Autodesk Inventor part; units mm, degrees
ref_plane "YZ Plane" through (0, 0, 0) normal (1, 0, 0) x (0, 1, 0)
ref_plane "XZ Plane" through (0, 0, 0) normal (0, 1, 0) x (-1, 0, 0)
ref_plane "XY Plane" through (0, 0, 0) normal (0, 0, 1) x (1, 0, 0)
sketch "Skizze1" plane through (0, 0, 0) normal (0, 0, 1) x (1, 0, 0)
  line L0 (0, 12.3) -> (8.8, 12.3)
  line L1 (0, 12.3) -> (0, 0)
  line L2 (0, 0) -> (8.8, 0)
  line L3 (8.8, 0) -> (8.8, 12.3)
  circle A0 centre (5.18, 3.55) radius 1.25
  circle A1 centre (5.18, 3.55) radius 1.25
  line L4 (0, 12.3) -> (8.8, 12.3)
  line L5 (8.8, 12.3) -> (8.8, 0)
  line L6 (8.8, 0) -> (0, 0)
  line L7 (0, 0) -> (0, 12.3)
  dimension "d35" = 8.8
  dimension "d36" = 5.18
extrude "Extrusion1" add sketch "Skizze1" along normal blind 9.8
sketch "Skizze2" plane through (8.8, 0, 0) normal (1, 0, 0) x (0, 0, -1)
  line L0 (0, 0) -> (-9.8, 0)
  line L1 (0, 0) -> (0, 12.3)
  line L2 (0, 12.3) -> (-9.8, 12.3)
  line L3 (-4.8, 6.1) -> (0, 6.1)
  line L4 (0, 6.1) -> (0, 0)
  line L5 (0, 0) -> (-4.8, 0)
  line L6 (-4.8, 0) -> (-4.8, 6.1)
  dimension "d2" = 6.2
  dimension "d3" = 4.8
  dimension "d4" = 6.1
extrude "Extrusion2" cut sketch "Skizze2" against normal blind 9.8
sketch "Skizze3" plane through (8.8, 0, 9.8) normal (1, 0, 0) x (0, 0, -1)
  line L0 (9.8, 6.1) -> (9.8, 12.3)
  line L1 (9.8, 12.3) -> (0, 12.3)
  point P0 (9.8, 0)
  point P1 (6.1, 8.6)
  dimension "d7" = 3.7
  dimension "d8" = 3.7
hole "Hole1" at (8.8, 8.6, 3.7) direction (-1, 0, 0) diameter 2.013 end through all
sketch "Skizze4" plane through (0, 0, 9.8) normal (0, 0, 1) x (1, 0, 0)
  circle A0 centre (5.18, 3.55) radius 1.25
  circle A1 centre (5.18, 3.55) radius 1.25
extrude "Extrusion3" add sketch "Skizze4" against normal blind 5
sketch "Skizze5" plane through (0, 0, 9.8) normal (0, 0, 1) x (1, 0, 0)
  line L0 (8.8, 0) -> (0, 0)
  line L1 (8.8, 12.3) -> (8.8, 0)
  point P0 (5.2, 3.55)
  dimension "d18" = 3.6
  dimension "d19" = 3.55
hole "Hole2" at (5.2, 3.55, 9.8) direction (0, 0, -1) diameter 2.013 depth 8 tip angle 118
fillet "Rundung1" radius 0.2 1 edges at (0, 12.3, 4.9)
fillet "Rundung2" radius 0.1 18 edges at (0, 9.1, 0) (0.0586, 12.2414, 0) (4.5, 12.3, 0) (0, 6.1, 2.4) (0, 3.05, 4.8) (4.4, 0, 4.8) (4.4, 6.1, 4.8) (4.4, 6.1, 0) (8.8, 9.2, 0) (8.8, 3.05, 4.8) (8.8, 0, 7.3) (0, 0, 7.3) (8.8, 12.3, 4.9) (8.8, 6.15, 9.8) (4.4, 0, 9.8) (0, 6.05, 9.8) (0.0586, 12.2414, 9.8) (4.5, 12.3, 9.8)
sketch "Skizze6" plane through (0.1, 0, 9.7) normal (0, -1, 0) x (1, 0, 0)
  line L0 (8.6, 0.1) -> (0, 0.1)
  line L1 (-0.1, 0) -> (-0.1, -4.8)
  line L2 (8.7, -4.8) -> (8.7, 0)
  line L3 (1.699, 0.1) -> (6.901, 0.1)
  line L4 (6.901, 0.1) -> (6.901, -0.1)
  line L5 (6.901, -0.1) -> (1.699, -0.1)
  line L6 (1.699, -0.1) -> (1.699, 0.1)
  point P0 (-0.1, -9.7)
  dimension "d30" = 0.2
  dimension "d31" = 1.799
  dimension "d32" = 1.799
extrude "Extrusion4" cut sketch "Skizze6" against normal blind 12.5
properties part number "3. Leiterplattenhalter_Rechts"
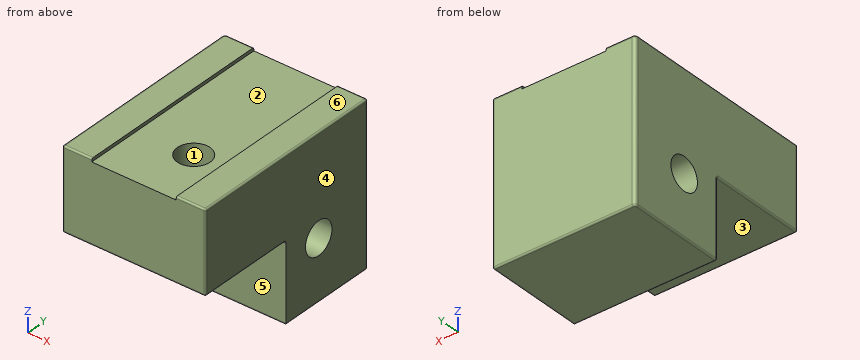
The model under review builds one solid part; all positions refer to its coordinate system, in mm. Face numbers are marked on the shaded views. A direction names the side the tool comes from. Round coordinates to 2 decimals unless told otherwise and drop trailing zeros. Order: outer loops, then holes, each group sorted by start corner. A loop starts at its lowest first (then second) coordinate and runs counter-clockwise, first axis right, second up. Notation, with made-up numbers: (12, 21.5) -> (67, 21.5) arc R19 cw to (67, 55.5) -> close; hole circle Ø1 at (-37.75, 5). An arc over 180 degrees is marked (long way). One line per item, written item: value. Start each with the question number.
Q1. Clearance check with flat-ended pins moving along their axes: pin 1 Ø4 at (x, y) = (4, 7) entering from +Z; pin 2 Ø5 at (x, z) = (5.5, 1.5) entering from -Y; pin 3 Ø4.5 at (x, y) = (2.5, 2.5) entering from -Z. State where each tip first meets the part, or that it passes through.
Q2. Machinability: for the marked faces 5 and 6, which of the approach directions +Z, -Z, +X, -X, +Y, -Y give a long, thin tool a straight path to every point of the face, cutting with its end or side? Answer none if there is none.
Q3. Take a section at C-C (y = 3.55). Write out the cut boundary in (x, z), and give its area (3 significant figures).
Q4. Take a section at A-A (x = 5.2). Write out the cut boundary in (y, z), and give its area (3 significant figures).
Q5. Take a section at B-B (z = 3.7). Write out the cut boundary in (x, y).
Q6. Mouldability with a two-part tool opening along X and no side actions: class the marked faces 1, 2, 3 and 4 as released by +X, released by -X, zero draft, split by the parting line, or undercut.
Q7. Wall thickness on line 1 (X direction, y = 3.55, z = 7.55); line 2 (Y direction, x = 2.25, z = 3.7); line 3 (Z direction, x = 3.75, y = 8.6): over which ranges is each line inside the solid? List them lowest first.
Q8. Take a section at D-D (x = 8.25). Write out the cut boundary in (y, z), and give its area (3 significant figures).
Reported:
1. pin 1: stops at z = 9.6
1. pin 2: stops at y = 6.1
1. pin 3: stops at z = 4.8
2. face 5: -Z, +X, -X, -Y
2. face 6: +Z, +X, -X, +Y, -Y
3. outline: (0, 4.9) arc R0.1 ccw to (0.1, 4.8) -> (4.19, 4.8) -> (4.19, 9.6) -> (1.8, 9.6) -> (1.8, 9.8) -> (0.1, 9.8) arc R0.1 ccw to (0, 9.7) -> close; (6.21, 4.8) -> (8.7, 4.8) arc R0.1 ccw to (8.8, 4.9) -> (8.8, 9.7) arc R0.1 ccw to (8.7, 9.8) -> (7, 9.8) -> (7, 9.6) -> (6.21, 9.6) -> close
3. area: 33.3 mm2
4. outline: (0, 4.9) arc R0.1 ccw to (0.1, 4.8) -> (2.54, 4.8) -> (2.54, 9.6) -> (0, 9.6) -> close; (4.56, 4.8) -> (6, 4.8) arc R0.1 cw to (6.1, 4.7) -> (6.1, 0.1) arc R0.1 ccw to (6.2, 0) -> (12.2, 0) arc R0.1 ccw to (12.3, 0.1) -> (12.3, 9.6) -> (4.56, 9.6) -> close; hole circle Ø2.01 at (8.6, 3.7)
4. area: 76.0 mm2
5. outline: (0, 6.2) arc R0.1 ccw to (0.1, 6.1) -> (8.8, 6.1) -> (8.8, 7.59) -> (0, 7.59) -> close; (0, 9.61) -> (8.8, 9.61) -> (8.8, 12.2) arc R0.1 ccw to (8.7, 12.3) -> (0.2, 12.3) arc R0.2 ccw to (0, 12.1) -> close
6. face 1: undercut
6. face 2: undercut
6. face 3: zero draft
6. face 4: released by +X
7. line 1: x = 0 to 4.19, 6.21 to 8.8
7. line 2: y = 6.1 to 7.59, 9.61 to 12.3
7. line 3: z = 0 to 2.69, 4.71 to 9.6
8. outline: (0, 4.9) arc R0.1 ccw to (0.1, 4.8) -> (6, 4.8) arc R0.1 cw to (6.1, 4.7) -> (6.1, 0.1) arc R0.1 ccw to (6.2, 0) -> (12.2, 0) arc R0.1 ccw to (12.3, 0.1) -> (12.3, 9.7) arc R0.1 ccw to (12.2, 9.8) -> (0.1, 9.8) arc R0.1 ccw to (0, 9.7) -> close; hole circle Ø2.01 at (8.6, 3.7)
8. area: 88.1 mm2
